from build123d import *

# Parameters (mm, degrees)
SKETCH_1_R          = 10
EXTRUDE_1_DEPTH     = 30
SKETCH_2_R          = 4.5
CUT_EXTRUDE_1_DEPTH = 30
EXTRUDE_START       = 4.5
EXTRUDE_2_DEPTH     = 66.3
EXTRUDE_3_DEPTH     = 5
EXTRUDE_START_2     = -5
EXTRUDE_4_DEPTH     = 5
SKETCH_6_R          = 4.5
CUT_EXTRUDE_2_DEPTH = 27
SKETCH_17_R         = 5
EXTRUDE_9_DEPTH     = 45


with BuildPart() as part:
    # 草图1 → 凸台-拉伸1 (new body)
    with BuildSketch(Plane.XY):
        Circle(SKETCH_1_R)
    extrude(amount=EXTRUDE_1_DEPTH)

    # 草图2 → 切除-拉伸1 (cut)
    with BuildSketch(Plane.XY.offset(30)):
        Circle(SKETCH_2_R)
    extrude(amount=-CUT_EXTRUDE_1_DEPTH, mode=Mode.SUBTRACT)

    # 草图3 → 凸台-拉伸2 (add)
    with BuildSketch(Plane(origin=(0, 0, 0), x_dir=(1, 0, 0), z_dir=(0, 1, 0)).offset(EXTRUDE_START)):
        Polygon((0, -19.5), (7, -19.5), (7, -24.5), (-7, -24.5), (-7, -19.5), align=None)
        Polygon((0, -10.5), (7, -10.5), (7, -5.5), (-7, -5.5), (-7, -10.5), align=None)
    extrude(amount=EXTRUDE_2_DEPTH)

    # 草图4 → 凸台-拉伸3 (add)
    with BuildSketch(Plane(origin=(0, 0, 5.5), x_dir=(-1, 0, 0), z_dir=(0, 0, -1))):
        with BuildLine():
            Line((-7, 70.8), (7, 70.8))
            ThreePointArc((7, 70.8), (0, 77.8), (-7, 70.8))
        make_face()
    extrude(amount=-EXTRUDE_3_DEPTH)

    # 草图5 → 凸台-拉伸4 (add)
    with BuildSketch(Plane.XY.offset(24.5).offset(EXTRUDE_START_2)):
        with BuildLine():
            Line((-7, 70.8), (7, 70.8))
            ThreePointArc((7, 70.8), (0, 77.8), (-7, 70.8))
        make_face()
    extrude(amount=EXTRUDE_4_DEPTH)

    # 草图6 → 切除-拉伸2 (cut)
    with BuildSketch(Plane(origin=(0, 0, 5.5), x_dir=(-1, 0, 0), z_dir=(0, 0, -1))):
        with Locations((0, 70.8)):
            Circle(SKETCH_6_R)
    extrude(amount=-CUT_EXTRUDE_2_DEPTH, mode=Mode.SUBTRACT)

    # 草图15 → 旋转1 (revolve)
    with BuildSketch(Plane.XY.offset(15)):
        Polygon((-4.417472119, -0.857869498), (-5.942573449, 6.99541427), (-30.974915458, 2.134153781), (-29.449814128, -5.719129986), align=None)
    revolve(axis=Axis((-4.417472119, -0.857869498, 15), (-0.9816604709485747, -0.1906376662074486, 0)))

    # 草图17 → 凸台-拉伸9 (add)
    with BuildSketch(Plane(origin=(-29.449814128, -5.719129986, 0), x_dir=(0, 0, 1), z_dir=(-0.9816604709485748, -0.19063766620744863, 0))):
        with Locations(Location((15, 0, 0), (0, 0, 270))):
            Circle(SKETCH_17_R)
    extrude(amount=EXTRUDE_9_DEPTH)


solid = part.part
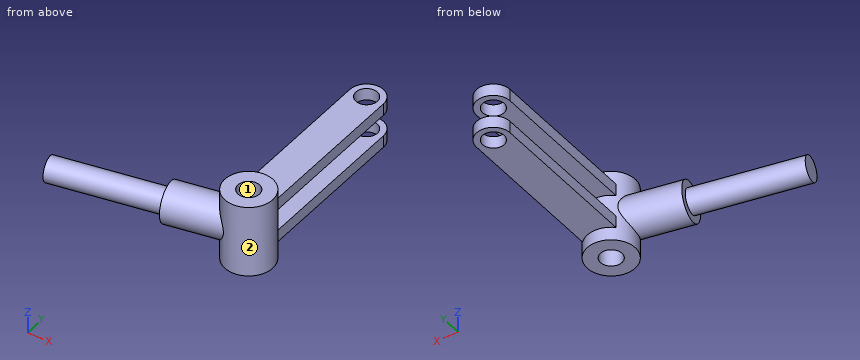
The listing builds one solid part. Answer for the finished solid, in the listing's coordinates (mm). Face numbers are marked on the shaded views. A direction names the side the tool comes from. Give positions to 0.01 mm unless a question says otherwise; leave off trailing zeros. Write each loop counter-clockwise with the first axis right and the second up, starting at its lowest first coordinate (ties: lowest second). Pieces come first, ordered by that corner, then holes.
1) Given P1, Ø10, axis at y = 40, z = 11.5, coming from the +X side; P2, Ø4, axis at y = 13.5, z = 21, coming from the -X side; P3, Ø7, axis at x = -1, y = 44.5, coming from the -Z side; P4, Ø8, axis at x = 0, y = 70.8, coming from the +Z side, each flat-ended and moving along its own axis, determine where each tip first touches the part or whether it passes through.
2) Section C-C (z = 27.5) is taken. Write down the section's boundary in (x, y), and give its area (3 significant figures).
3) Find the intervals of material crossed by L1, parallel to Y at x = 0, z = 22.6; L2, parallel to Z at x = -6, y = 35; L3, parallel to X at y = 25.5, z = 9, in increasing order.
4) Section B-B (x = 0) is taken. Write down the section's boundary in (y, z).
5) A tool of negligible diameter and unlimited length cuts with its end or side. For the marked faces 1 and 2, from which of +Z, -Z, +X, -X, +Y, -Y can it reach the whole face along a straight path? Write none if from no direction.
6) Section A-A (y = 61) is taken. Write down the section's boundary in (x, z), and give its area (3 significant figures).
Response:
1. P1: stops at x = 7
1. P2: stops at x = -7
1. P3: stops at z = 5.5
1. P4: passes through
2. outline: circle Ø20 at (0, 0); hole circle Ø9 at (0, 0)
2. area: 251 mm2
3. L1: y = -10 to -4.5, 4.5 to 66.3, 75.3 to 77.8
3. L2: z = 5.5 to 10.5, 19.5 to 24.5
3. L3: x = -7 to 7
4. outline: (-10, 0) - (-4.5, 0) - (-4.5, 30) - (-10, 30) - close; (4.5, 0) - (10, 0) - (10, 5.5) - (66.3, 5.5) - (66.3, 10.5) - (10, 10.5) - (10, 19.5) - (66.3, 19.5) - (66.3, 24.5) - (10, 24.5) - (10, 30) - (4.5, 30) - close; (75.3, 5.5) - (77.8, 5.5) - (77.8, 10.5) - (75.3, 10.5) - close; (75.3, 19.5) - (77.8, 19.5) - (77.8, 24.5) - (75.3, 24.5) - close
5. face 1: +Z, -Z
5. face 2: none
6. outline: (-7, 5.5) - (7, 5.5) - (7, 10.5) - (-7, 10.5) - close; (-7, 19.5) - (7, 19.5) - (7, 24.5) - (-7, 24.5) - close
6. area: 140 mm2
